```python
from build123d import *

# Parameters (mm, degrees)
F2_R         = 15
F2_R_2       = 2
F2_R_3       = 7.5
F2_R_4       = 4.9
F3_DEPTH     = 11
F4_DEPTH     = 9
F5_DEPTH     = 18.5
F2_R_5       = 16
F10_DEPTH    = 1
F11_START    = 9
F10_FACE_R   = 16
F10_FACE_R_2 = 15
F11_DEPTH    = 1
F12_DEPTH    = 12


with BuildPart() as f3:
    # F2 (on Top) → F3 (new body)
    with BuildSketch(Plane.XY):
        Circle(F2_R)
        with Locations((-6.6125840883, -9.1014411867)):
            Circle(F2_R_2, mode=Mode.SUBTRACT)
        with Locations((-10.6993858083, -3.4764411867)):
            Circle(F2_R_2, mode=Mode.SUBTRACT)
        with Locations((0, -11.25)):
            Circle(F2_R_2, mode=Mode.SUBTRACT)
        with Locations((6.6125840883, -9.1014411867)):
            Circle(F2_R_2, mode=Mode.SUBTRACT)
        with Locations((10.6993858083, -3.4764411867)):
            Circle(F2_R_2, mode=Mode.SUBTRACT)
        with Locations((-10.6993858083, 3.4764411867)):
            Circle(F2_R_2, mode=Mode.SUBTRACT)
        with Locations((-6.6125840883, 9.1014411867)):
            Circle(F2_R_2, mode=Mode.SUBTRACT)
        Circle(F2_R_3, mode=Mode.SUBTRACT)
        with Locations((10.6993858083, 3.4764411867)):
            Circle(F2_R_2, mode=Mode.SUBTRACT)
        with Locations((0, 11.25)):
            Circle(F2_R_2, mode=Mode.SUBTRACT)
        with Locations((6.6125840883, 9.1014411867)):
            Circle(F2_R_2, mode=Mode.SUBTRACT)
        Circle(F2_R_3)
        Circle(F2_R_4, mode=Mode.SUBTRACT)
        Circle(F2_R_4)
        with BuildLine():
            ThreePointArc((-2.2847319318, -2.45), (-3.35, 0), (-2.2847319318, 2.45))
            Line((-2.2847319318, 2.45), (2.2847319318, 2.45))
            ThreePointArc((2.2847319318, 2.45), (3.35, 0), (2.2847319318, -2.45))
            Line((2.2847319318, -2.45), (-2.2847319318, -2.45))
        make_face(mode=Mode.SUBTRACT)
    extrude(amount=F3_DEPTH)

    # F2 (on Top) → F4 (join)
    with BuildSketch(Plane.XY):
        Circle(F2_R_3)
        Circle(F2_R_4, mode=Mode.SUBTRACT)
        Circle(F2_R_4)
        with BuildLine():
            ThreePointArc((-2.2847319318, -2.45), (-3.35, 0), (-2.2847319318, 2.45))
            Line((-2.2847319318, 2.45), (2.2847319318, 2.45))
            ThreePointArc((2.2847319318, 2.45), (3.35, 0), (2.2847319318, -2.45))
            Line((2.2847319318, -2.45), (-2.2847319318, -2.45))
        make_face(mode=Mode.SUBTRACT)
    extrude(amount=F4_DEPTH)

    # F2 (on Top) → F5 (join)
    with BuildSketch(Plane.XY):
        Circle(F2_R_4)
        with BuildLine():
            ThreePointArc((-2.2847319318, -2.45), (-3.35, 0), (-2.2847319318, 2.45))
            Line((-2.2847319318, 2.45), (2.2847319318, 2.45))
            ThreePointArc((2.2847319318, 2.45), (3.35, 0), (2.2847319318, -2.45))
            Line((2.2847319318, -2.45), (-2.2847319318, -2.45))
        make_face(mode=Mode.SUBTRACT)
    extrude(amount=F5_DEPTH)

    # F6 (on Front) → F7 (revolve)
    with BuildSketch(Plane.XZ):
        Polygon((5.15, 17.75), (4.9, 18.5), (4.9, 17), align=None)
    revolve(axis=Axis((0, 0, 8.7542282417), (0, 0, 1)))

    # F2 (on Top) → F10 (join)
    with BuildSketch(Plane.XY):
        Circle(F2_R_5)
        Circle(F2_R, mode=Mode.SUBTRACT)
    extrude(amount=F10_DEPTH)

    # F2 (on Top) + F10_face (on face) → F11 (join)
    with BuildSketch(Plane.XY.offset(F11_START)):
        Circle(F2_R)
        with Locations((-6.6125840883, -9.1014411867)):
            Circle(F2_R_2, mode=Mode.SUBTRACT)
        with Locations((-10.6993858083, -3.4764411867)):
            Circle(F2_R_2, mode=Mode.SUBTRACT)
        with Locations((0, -11.25)):
            Circle(F2_R_2, mode=Mode.SUBTRACT)
        with Locations((6.6125840883, -9.1014411867)):
            Circle(F2_R_2, mode=Mode.SUBTRACT)
        with Locations((10.6993858083, -3.4764411867)):
            Circle(F2_R_2, mode=Mode.SUBTRACT)
        with Locations((-10.6993858083, 3.4764411867)):
            Circle(F2_R_2, mode=Mode.SUBTRACT)
        with Locations((-6.6125840883, 9.1014411867)):
            Circle(F2_R_2, mode=Mode.SUBTRACT)
        Circle(F2_R_3, mode=Mode.SUBTRACT)
        with Locations((10.6993858083, 3.4764411867)):
            Circle(F2_R_2, mode=Mode.SUBTRACT)
        with Locations((0, 11.25)):
            Circle(F2_R_2, mode=Mode.SUBTRACT)
        with Locations((6.6125840883, 9.1014411867)):
            Circle(F2_R_2, mode=Mode.SUBTRACT)
    with BuildSketch(Plane.XY.offset(1).offset(F11_START)):
        Circle(F10_FACE_R)
        Circle(F10_FACE_R_2, mode=Mode.SUBTRACT)
    extrude(amount=F11_DEPTH)

    # F2 (on Top) → F12 (join)
    with BuildSketch(Plane.XY):
        Circle(F2_R_3)
        Circle(F2_R_4, mode=Mode.SUBTRACT)
    extrude(amount=F12_DEPTH)


solid = f3.part
```
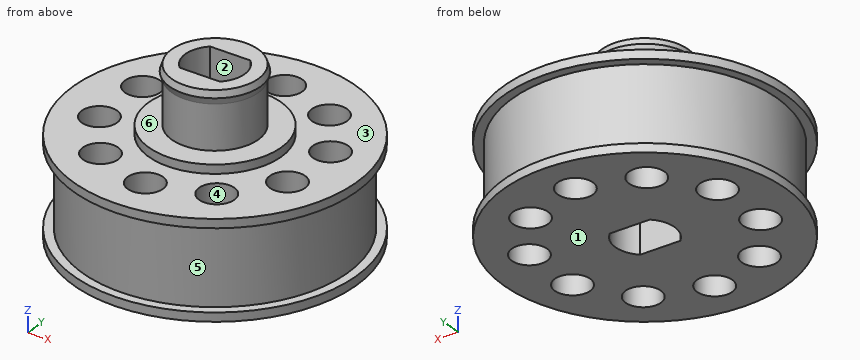
Verification items for the finished model (mm, model axes). Face numbers are marked on the shaded views. A direction names the side the tool comes from. Round coordinates to 2 decimals unless told otherwise and drop trailing zeros. Order: outer loops, then holes, each group sorted by start corner. A loop starts at its lowest first (then second) coordinate and runs counter-clockwise, first axis right, second up. Notation, with made-up numbers: (32.5, -9) -> (80.5, -9) arc R20 ccw to (80.5, 7) -> close; hole circle Ø7 at (-30, 26). An arc over 180 degrees is marked (long way). Put each result on its own line as item: value. Start each with the question number.
(1) Section check C-C (x = 6). Enter the section's corners in (y, z).
(2) Section check B-B (z = 3.25). State how many separate pieces and enclosed holes the cut face has, then the cut area to 3 significant figures.
(3) Draft check along Y on the marked faces 4, 5 and 6. Enter one of: +Y half, -Y half, draft (parallel to the pull), parting line (faces both ways), or undercut.
(4) Section check A-A (y = 0). Enter the section's corners in (x, z), then the cut area to 3 significant figures.
(5) Tool access check on the marked faces 1, 2 and 3. Record the directions out of +Z, -Z, +X, -X, +Y, -Y that give a thin tool (end or side, any length) a straight path to the whole face; none if there is none.
(6) Depth check by flat-ended pin: pin 1 Ø8 at (x, y) = (12, 5.5) entering from +Z; pin 2 Ø2 at (x, z) = (-10, 5) entering from -Y; pin 3 Ø3.5 at (x, z) = (1, 6) entering from +Y; pin 4 Ø3 at (x, y) = (0, -11.25) entering from -Z. Enter the tip coordinate at first touch or a pass-through.
(7) Material ranges on line 1 along Y through (x, z) = (0, 2.5); line 2 along Y through (x, z) = (-5, 5); line 3 along Y through (x, z) = (-1.5, 6.5), recorded low to high.
Completed:
1. outline: (-14.83, 0) -> (-11.01, 0) -> (-11.01, 11) -> (-14.83, 11) -> (-14.83, 10) -> (-13.75, 10) -> (-13.75, 1) -> (-14.83, 1) -> close; (-7.2, 0) -> (7.2, 0) -> (7.2, 11) -> (4.5, 11) -> (4.5, 12) -> (-4.5, 12) -> (-4.5, 11) -> (-7.2, 11) -> close; (11.01, 0) -> (14.83, 0) -> (14.83, 1) -> (13.75, 1) -> (13.75, 10) -> (14.83, 10) -> (14.83, 11) -> (11.01, 11) -> close
2. separate pieces: 1
2. enclosed holes: 11
2. area: 552 mm2
3. face 4: undercut
3. face 5: parting line
3. face 6: draft
4. outline: (-16, 0) -> (-3.35, 0) -> (-3.35, 18.5) -> (-4.9, 18.5) -> (-5.15, 17.75) -> (-4.9, 17) -> (-4.9, 12) -> (-7.5, 12) -> (-7.5, 11) -> (-16, 11) -> (-16, 10) -> (-15, 10) -> (-15, 1) -> (-16, 1) -> close; (3.35, 0) -> (16, 0) -> (16, 1) -> (15, 1) -> (15, 10) -> (16, 10) -> (16, 11) -> (7.5, 11) -> (7.5, 12) -> (4.9, 12) -> (4.9, 17) -> (5.15, 17.75) -> (4.9, 18.5) -> (3.35, 18.5) -> close
4. area: 289 mm2
5. face 1: -Z, +X, -X, +Y, -Y
5. face 2: +Z, -Z
5. face 3: +Z
6. pin 1: stops at z = 11
6. pin 2: stops at y = -12
6. pin 3: stops at y = 15
6. pin 4: passes through
7. line 1: y = -15 to -13.25, -9.25 to -2.45, 2.45 to 9.25, 13.25 to 15
7. line 2: y = -14.14 to -10.28, -7.92 to 7.92, 10.28 to 14.14
7. line 3: y = -14.92 to -12.57, -9.93 to -2.45, 2.45 to 9.93, 12.57 to 14.92
